Work out the finished part from the listing and answer in its coordinate system (mm). A direction names the side the tool comes from. Round coordinates to 2 decimals unless told otherwise and drop trailing zeros. Order: outer loops, then holes, each group sorted by start corner. A loop starts at its lowest first (then second) coordinate and runs counter-clockwise, first axis right, second up.
Autodesk Inventor part; units mm, degrees
ref_plane "YZ Plane" through (0, 0, 0) normal (1, 0, 0) x (0, 1, 0)
ref_plane "XZ Plane" through (0, 0, 0) normal (0, 1, 0) x (-1, 0, 0)
ref_plane "XY Plane" through (0, 0, 0) normal (0, 0, 1) x (1, 0, 0)
sketch "Sketch1" plane through (0, 0, 0) normal (0, 0, 1) x (1, 0, 0)
  circle A0 centre (0, 0) radius 2
  dimension "d0" = 4
extrude "Extrusion1" add sketch "Sketch1" along normal blind 1.25
fillet "Fillet1" radius 0.5 1 edges at (-2, 0, 0)
fillet "Fillet2" radius 0.75 1 edges at (-2, 0, 1.25)
sketch "Sketch2" plane through (0, 0, 1.25) normal (0, 0, 1) x (1, 0, 0)
  line L0 (-1.25, -0.2499) -> (-1.25, 0.2501)
  line L1 (-1.25, 0.2501) -> (-0.25, 0.2501)
  line L2 (-0.25, 0.2501) -> (-0.25, 1.2501)
  line L3 (-0.25, 1.2501) -> (0.25, 1.2501)
  line L4 (0.25, 1.2501) -> (0.25, 0.2501)
  line L5 (0.25, 0.2501) -> (1.25, 0.2501)
  line L6 (1.25, 0.2501) -> (1.25, -0.2499)
  line L7 (1.25, -0.2499) -> (0.25, -0.2499)
  line L8 (0.25, -0.2499) -> (0.25, -1.2499)
  line L9 (0.25, -1.2499) -> (-0.25, -1.2499)
  line L10 (-0.25, -1.2499) -> (-0.25, -0.2499)
  line L11 (-0.25, -0.2499) -> (-1.25, -0.2499)
  dimension "d24" = 0.5
  dimension "d27" = 0.5
  dimension "d28" = 0.5
  dimension "d29" = 0.5
  dimension "d30" = 1
  dimension "d31" = 1
  dimension "d32" = 1
  dimension "d33" = 1
  dimension "d34" = 1
  dimension "d35" = 1
extrude "Extrusion2" cut sketch "Sketch2" against normal blind 1
sketch "Sketch3" plane through (0, 0, 0) normal (0, 0, -1) x (-1, 0, 0)
  circle A0 centre (0, 0) radius 1.5
  circle A1 centre (0, 0) radius 1
  dimension "d19" = 2
extrude "Extrusion3" add sketch "Sketch3" along normal blind 8 contours A1
chamfer "Chamfer3" distance 0.5 angle 45 4 edges at (-1.25, 0.0001, 0.25) (0, 1.2501, 0.25) (0, -1.2499, 0.25) (1.25, 0.0001, 0.25)
thread "Thread2"
properties part number "screw_M2_8"
Item 1: Find the intervals of material crossed by line 1 along Z through (x, y) = (-0.05, -0.7); line 2 along Y through (x, z) = (-0.05, -5.25); line 3 along Z through (x, y) = (-0.35, -1), in increasing order.
Item 2: Given pin 1 (0.8 mm diameter, centred on x = -0.5, z = 1, fed in from +Y); pin 2 (1.6 mm diameter, centred on x = -0.5, y = 0, fed in from +Z), each flat-ended and moving along its own axis, determine where each tip first touches the part or whether it passes through.
Item 3: A tool of negligible diameter and unlimited length cuts with its end or side. For faces 1 (the face through (0.25, -1, 1)), 2 (the face through (-0.6, -0.6, 1.25)), from which of +Z, -Z, +X, -X, +Y, -Y can it reach the whole face along a straight path? Write none if from no direction.
Item 4: For a pull along Y with two mould halves and no side action, classify faces 3 (the face through (-0.6, 0.6, 1.25)), 4 (the face through (1, 0.25, 1)), 5 (the face through (0, 1, -4)) as released by +Y, released by -Y, zero draft, split by the parting line, or undercut.
Item 5: Find section A-A (z = -3.25). Write down the section's boundary in (x, y), plus the area to 3 significant figures.
Model answer:
1. line 1: z = -8 to 0.25
1. line 2: y = -1 to 1
1. line 3: z = 0 to 1.25
2. pin 1: stops at y = 1.96
2. pin 2: stops at z = 1.25
3. face 1: +Z
3. face 2: +Z, +X, -X, +Y, -Y
4. face 3: zero draft
4. face 4: undercut
4. face 5: split by the parting line
5. outline: circle Ø2 at (0, 0)
5. area: 3.14 mm2
